Could you check a few things on this drawing? It's one solid part, dimensions in mm from its lowest x, y, z. A direction names the side the tool comes from. Round coordinates to 2 decimals unless told otherwise and drop trailing zeros. Write each loop counter-clockwise with the first axis right and the second up, starting at its lowest first coordinate (ties: lowest second). Pieces come first, ordered by that corner, then holes. Notation, with made-up numbers: (40, -22.75) -> (79, -22.75) arc R11 cw to (79, -2.75) -> close; hole circle Ø3 at (-29, 55.25). An arc over 180 degrees is marked (long way). Return JSON: item names as keys, results as strings.
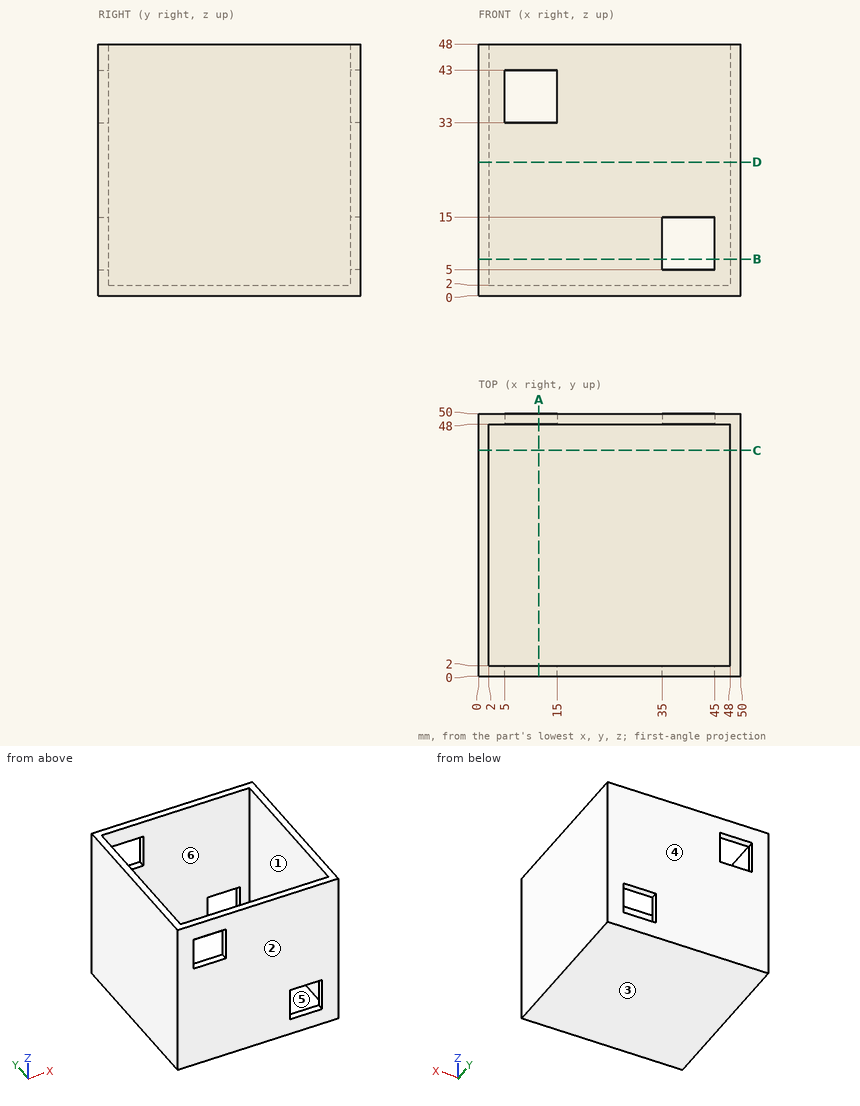
1) I want a section at D-D, the plane z = 25.5. Please give me the cut outline in (x, y).
Return value:
{"outline": "(0, 0) -> (50, 0) -> (50, 50) -> (0, 50) -> close; hole (2, 2) -> (48, 2) -> (48, 48) -> (2, 48) -> close"}
2) Thinking about a two-plate mould opening in Y: for the marked faces 3, 4, 5 and 6, which applies, pulls with the +Y half, pulls with the -Y half, needs draft (parallel to the pull), parting line crosses it, or undercut?
Return value:
{"face 3": "needs draft", "face 4": "pulls with the +Y half", "face 5": "undercut", "face 6": "undercut"}
3) Will this pin go through, and if not, where does the flat tip stop? pin 1 Ø14 at (x, y) = (27.5, 17.5) entering from +Z.
Return value:
{"pin 1": "z = 2"}
4) I want a section at C-C, the plane y = 43. Please give me the cut outline in (x, z).
Return value:
{"outline": "(0, 0) -> (50, 0) -> (50, 48) -> (48, 48) -> (48, 2) -> (2, 2) -> (2, 48) -> (0, 48) -> close"}
5) For the marked faces 1 and 2, which set-ups out of +Z, -Z, +X, -X, +Y, -Y let a thin tool reach every point of the face, with its end or its side?
Return value:
{"face 1": "+Z", "face 2": "+Z, -Z, +X, -X, -Y"}
6) If I drill on probe 1 along X at (y, z) = (41, 6.5); probe 2 along Z at (x, y) = (39.5, 26.5), over which ranges is the centre line in solid material (lowest first)? Write a range as [from, to].
Return value:
{"probe 1": "[0, 2], [48, 50]", "probe 2": "[0, 2]"}
7) I want a section at B-B, the plane z = 7. Please give me the cut outline in (x, y).
Return value:
{"outline": "(0, 0) -> (35, 0) -> (35, 2) -> (2, 2) -> (2, 48) -> (35, 48) -> (35, 50) -> (0, 50) -> close; (45, 0) -> (50, 0) -> (50, 50) -> (45, 50) -> (45, 48) -> (48, 48) -> (48, 2) -> (45, 2) -> close"}
8) I want a section at A-A, the plane x = 11.5. Please give me the cut outline in (y, z), and give its area (3 significant figures).
Return value:
{"outline": "(0, 0) -> (50, 0) -> (50, 33) -> (48, 33) -> (48, 2) -> (2, 2) -> (2, 33) -> (0, 33) -> close; (0, 43) -> (2, 43) -> (2, 48) -> (0, 48) -> close; (48, 43) -> (50, 43) -> (50, 48) -> (48, 48) -> close", "area": "244 mm²"}
